from build123d import *

# Parameters (mm, degrees)
SKETCH1_R                                        = 300
BOSS_EXTRUDE1_DEPTH                              = 15
CBORE_FOR_1_4_SOCKET_HEAD_CAP_SCREW1_D           = 7.14248
CBORE_FOR_1_4_SOCKET_HEAD_CAP_SCREW1_CBORE_D     = 11.1125
CBORE_FOR_1_4_SOCKET_HEAD_CAP_SCREW1_CBORE_DEPTH = 6.35


with BuildPart() as part:
    # Sketch1 → Boss-Extrude1 (new body)
    with BuildSketch(Plane(origin=(0, 0, 0), x_dir=(1, 0, 0), z_dir=(0, 1, 0))):
        with Locations(Location((0, 0, 0), (0, 0, 270))):
            Circle(SKETCH1_R)
    extrude(amount=BOSS_EXTRUDE1_DEPTH)

    # CBORE for 1/4 Socket Head Cap Screw1 (through all)
    with Locations(Plane.XZ):
        with Locations((-250, 0), (0, -250), (250, 0), (0, 250)):
            CounterBoreHole(CBORE_FOR_1_4_SOCKET_HEAD_CAP_SCREW1_D / 2, CBORE_FOR_1_4_SOCKET_HEAD_CAP_SCREW1_CBORE_D / 2, CBORE_FOR_1_4_SOCKET_HEAD_CAP_SCREW1_CBORE_DEPTH)


solid = part.part
Geometry: final body of the model. Coordinates: model frame, mm. Give positions to 0.01 mm unless a question says otherwise; leave off trailing zeros. Order: outer loops, then holes, each group sorted by start corner. A loop starts at its lowest first (then second) coordinate and runs counter-clockwise, first axis right, second up. Notation, with made-up numbers: (18, 43.25) - (37, 43.25) arc R20 ccw to (37, 56.25) - close; hole circle Ø9 at (-11.5, 70.5). An arc over 180 degrees is marked (long way). Use CSV: the item, a comma, the result in double quotes.
1. Contact query for flat-ended pins moving along their axis: pin 1 (1.5 mm diameter, centred on y = 2.5, z = -157, fed in from +X); pin 2 (12 mm diameter, centred on x = -249, z = -2, fed in from -Y); pin 3 (3.5 mm diameter, centred on x = 247.5, z = -1, fed in from -Y); pin 4 (3.5 mm diameter, centred on x = -1.5, z = -250, fed in from -Y). Output: stop coordinate, or through.
Answers below:
pin 1,"x = 256.1"
pin 2,"y = 0"
pin 3,"y = 6.35"
pin 4,"through"
2. Section query A-A (y = 11.5). Output: boundary loops of the cut face in (x, z), plus the area to 3 significant figures.
Answers below:
outline,"circle Ø600 at (0, 0); hole circle Ø7.14 at (-250, 0); hole circle Ø7.14 at (0, -250); hole circle Ø7.14 at (0, 250); hole circle Ø7.14 at (250, 0)"
area,"283,000 mm2"
3. Material intervals for line 1 along X through (y, z) = (9, 250); line 2 along X through (y, z) = (11.5, 4); line 3 along X through (y, z) = (6, 2), sorted ascending. Write a range as from..to.
Answers below:
line 1,"-165.83..-3.57, 3.57..165.83"
line 2,"-299.97..299.97"
line 3,"-299.99..-255.18, -244.82..244.82, 255.18..299.99"
4. Section query B-B (x = -187). Output: boundary loops of the cut face in (y, z), plus the area to 3 significant figures.
Answers below:
outline,"(0, -234.59) - (15, -234.59) - (15, 234.59) - (0, 234.59) - close"
area,"7,040 mm2"
5. Section query C-C (z = -133.5). Output: boundary loops of the cut face in (x, y), plus the area to 3 significant figures.
Answers below:
outline,"(-268.66, 0) - (268.66, 0) - (268.66, 15) - (-268.66, 15) - close"
area,"8,060 mm2"
